```python
from build123d import *

# Parameters (mm, degrees)
SKETCH1_W           = 141
SKETCH1_H           = 92
BOSS_EXTRUDE1_DEPTH = 2
SKETCH2_R           = 1.26
CUT_EXTRUDE1_DEPTH  = 10
FILLET1_R           = 1
SHELL1_T            = -1.5
FILLET2_R           = 1


with BuildPart() as part:
    # Sketch1 → Boss-Extrude1 (new body)
    with BuildSketch(Plane(origin=(0, 0, 0), x_dir=(1, 0, 0), z_dir=(0, 1, 0))):
        with Locations((70.5, 46)):
            Rectangle(SKETCH1_W, SKETCH1_H)
    extrude(amount=BOSS_EXTRUDE1_DEPTH)

    # Sketch2 → Cut-Extrude1 (cut)
    with BuildSketch(Plane.XZ):
        with Locations(Location((3, -3, 0), (0, 0, 270))):
            Circle(SKETCH2_R)
        with Locations(Location((138, -3, 0), (0, 0, 270))):
            Circle(SKETCH2_R)
        with Locations(Location((138, -89, 0), (0, 0, 270))):
            Circle(SKETCH2_R)
        with Locations(Location((3, -89, 0), (0, 0, 270))):
            Circle(SKETCH2_R)
    extrude(amount=-CUT_EXTRUDE1_DEPTH, mode=Mode.SUBTRACT)

    # Fillet1
    fillet1_edges = [part.edges().sort_by_distance(p)[0] for p in [
        (141, 2, -46),
        (70.5, 2, -92),
        (0, 2, -46),
        (70.5, 2, 0),
    ]]
    fillet(fillet1_edges, radius=FILLET1_R)

    # Shell1
    shell1_openings = [part.faces().sort_by_distance(p)[0] for p in [
        (70.5, 0, -46),
    ]]
    offset(amount=SHELL1_T, openings=shell1_openings, kind=Kind.INTERSECTION)

    # Fillet2
    # the kernel refuses this fillet: 1 mm, written as the material it takes off along each edge
    with BuildSketch(Plane(origin=(1, 1, -1), x_dir=(-1, 0, 0), z_dir=(0, 0, 1))) as fillet2_piece_1_section:
        Polygon((0, 0), (FILLET2_R, 0), (FILLET2_R, -FILLET2_R), (0, -FILLET2_R), align=None)
    fillet2_piece_1 = extrude(amount=FILLET2_R, mode=Mode.PRIVATE)
    fillet2_piece_1 = fillet2_piece_1 - Plane(origin=(1, 1, -1), x_dir=(0.7071067811865475, -0.7071067811865475, 0), z_dir=(0, 0, 1)) * Sphere(FILLET2_R, mode=Mode.PRIVATE)
    add(fillet2_piece_1, mode=Mode.SUBTRACT)
    with BuildSketch(Plane(origin=(1, 1, -91), x_dir=(-1, 0, 0), z_dir=(0, 0, -1))) as fillet2_piece_2_section:
        Polygon((0, 0), (FILLET2_R, 0), (FILLET2_R, FILLET2_R), (0, FILLET2_R), align=None)
    fillet2_piece_2 = extrude(amount=FILLET2_R, mode=Mode.PRIVATE)
    fillet2_piece_2 = fillet2_piece_2 - Plane(origin=(1, 1, -91), x_dir=(0.7071067811865475, -0.7071067811865475, 0), z_dir=(0, 0, -1)) * Sphere(FILLET2_R, mode=Mode.PRIVATE)
    add(fillet2_piece_2, mode=Mode.SUBTRACT)
    with BuildSketch(Plane(origin=(140, 1, -1), x_dir=(1, 0, 0), z_dir=(0, 0, 1))) as fillet2_piece_3_section:
        Polygon((0, 0), (FILLET2_R, 0), (FILLET2_R, FILLET2_R), (0, FILLET2_R), align=None)
    fillet2_piece_3 = extrude(amount=FILLET2_R, mode=Mode.PRIVATE)
    fillet2_piece_3 = fillet2_piece_3 - Plane(origin=(140, 1, -1), x_dir=(-0.7071067811865475, -0.7071067811865475, 0), z_dir=(0, 0, 1)) * Sphere(FILLET2_R, mode=Mode.PRIVATE)
    add(fillet2_piece_3, mode=Mode.SUBTRACT)
    with BuildSketch(Plane(origin=(140, 1, -91), x_dir=(0, 0, -1), z_dir=(1, 0, 0))) as fillet2_piece_4_section:
        Polygon((0, 0), (FILLET2_R, 0), (FILLET2_R, FILLET2_R), (0, FILLET2_R), align=None)
    fillet2_piece_4 = extrude(amount=FILLET2_R, mode=Mode.PRIVATE)
    fillet2_piece_4 = fillet2_piece_4 - Plane(origin=(140, 1, -91), x_dir=(0, -0.7071067811865475, 0.7071067811865475), z_dir=(1, 0, 0)) * Sphere(FILLET2_R, mode=Mode.PRIVATE)
    add(fillet2_piece_4, mode=Mode.SUBTRACT)
    with BuildSketch(Plane(origin=(141, -2.5, -92), x_dir=(0, 0, 1), z_dir=(0, 1, 0)), Plane(origin=(141, -2.5, 0), x_dir=(-1, 0, 0), z_dir=(0, 1, 0)), Plane(origin=(0, -2.5, -92), x_dir=(1, 0, 0), z_dir=(0, 1, 0))) as fillet2_piece_5:
        with BuildLine():
            CenterArc((FILLET2_R, -FILLET2_R), FILLET2_R, 90, 90)
            Line((0, -FILLET2_R), (0, 0))
            Line((0, 0), (FILLET2_R, 0))
        make_face()
    extrude(amount=3.5, mode=Mode.SUBTRACT)
    with BuildSketch(Plane(origin=(0, -2.5, 0), x_dir=(1, 0, 0), z_dir=(0, 1, 0))) as fillet2_piece_6:
        with BuildLine():
            CenterArc((FILLET2_R, FILLET2_R), FILLET2_R, 180, 90)
            Line((0, FILLET2_R), (0, 0))
            Line((0, 0), (FILLET2_R, 0))
        make_face()
    extrude(amount=3.5, mode=Mode.SUBTRACT)


solid = part.part
```
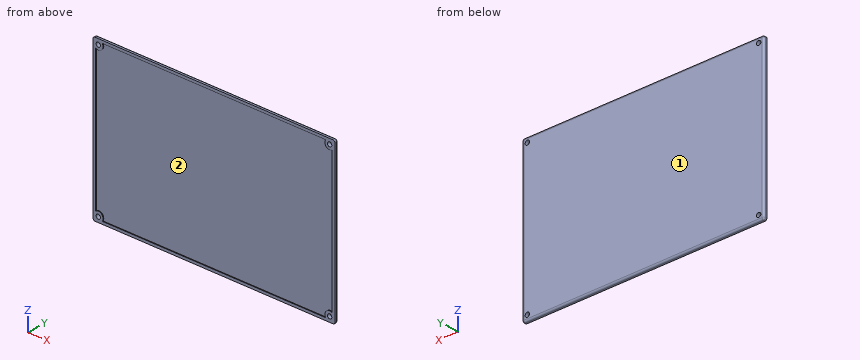
Check sheet for the modelled part. Datum: model origin and axes. Units: mm. Face numbers are marked on the shaded views. Round coordinates to 2 decimals unless told otherwise and drop trailing zeros. Loops run counter-clockwise (first coordinate to the right, second up) from the corner with the lowest first, then second, coordinate; pieces in that order, holes last. Notation, with made-up numbers: (-39, 25.25) -> (-7, 25.25) arc R12 cw to (-7, 29.25) -> close; hole circle Ø6 at (17, -32). An arc over 180 degrees is marked (long way). Write item = value, one per line. Start each with the question number.
1) Sectioned sample at B-B, the plane x = 37.5. Record the cut outline in (y, z), plus the area to 3 significant figures.
2) Gauge pin test, flat end, axial feed: pin 1 Ø5 at (x, z) = (54.5, -58) entering from -Y. Record the tip position at first contact, or that the pin passes through.
3) Release check for a two-part mould opening along Z. For the marked faces 1 and 2 record: released by +Z, released by -Z, zero draft, split by the parting line, or undercut.
4) Sectioned sample at A-A, the plane z = -64.5. Record the cut outline in (x, y).
5) Thickness scan on probe 1 along Z at (x, y) = (138, 0.45); probe 2 along X at (y, z) = (1.05, -89); probe 3 along X at (y, z) = (1.4, -89). Record the ranges inside material, lowest first.
Results are:
q1.outline = (0, -92) -> (1, -92) arc R1 ccw to (2, -91) -> (2, -1) arc R1 ccw to (1, 0) -> (0, 0) -> (0, -1.5) -> (0.5, -1.5) -> (0.5, -90.5) -> (0, -90.5) -> close
q1.area = 139 mm^2
q2.pin_1 = 0.5
q3.face_1 = zero draft
q3.face_2 = undercut
q4.outline = (0, 0) -> (1.5, 0) -> (1.5, 0.5) -> (139.5, 0.5) -> (139.5, 0) -> (141, 0) -> (141, 1) arc R1 ccw to (140, 2) -> (1, 2) arc R1 ccw to (0, 1) -> close
q5.probe_1 = -92 to -90.26, -87.74 to -86.24, -5.76 to -4.26, -1.74 to 0
q5.probe_2 = 0 to 1.74, 4.26 to 136.74, 139.26 to 141
q5.probe_3 = 0.08 to 1.74, 4.26 to 136.74, 139.26 to 140.92
